For this review, take the finished solid that the model builds, in its own axes (mm). A direction names the side the tool comes from. Coordinates: 2 decimals unless noted, no trailing zeros. Loops run counter-clockwise (first coordinate to the right, second up) from the corner with the lowest first, then second, coordinate; pieces in that order, holes last. Notation, with made-up numbers: (-15.75, 34.25) -> (7.25, 34.25) arc R6 ccw to (7.25, 39.25) -> close; hole circle Ø2 at (-35, 84). An arc over 180 degrees is marked (long way). Use a Markdown table: item, result.
from build123d import *

# Parameters (mm, degrees)
SKETCH_1_R               = 9.8
EXTRUDE_1_DEPTH          = 30
FILLET_1_R               = 0.5
CUT_EXTRUDE_1_DEPTH      = 34.046633746
CUT_EXTRUDE_1_DEPTH_BACK = 34.046633746
CUT_EXTRUDE_START        = -2
SKETCH_5_R               = 8
CUT_EXTRUDE_2_DEPTH      = 23
CHAMFER_1_SIZE           = 0.5
SKETCH_7_R               = 1.5
CUT_EXTRUDE_4_DEPTH      = 7
SKETCH_9_R               = 3
SKETCH_9_R_2             = 1.5
EXTRUDE_2_DEPTH          = 7
CHAMFER_2_SIZE           = 0.5


with BuildPart() as part:
    # Sketch 1 → Extrude 1 (new body)
    with BuildSketch(Plane(origin=(0, 0, 0), x_dir=(1, 0, 0), z_dir=(0, 1, 0))):
        with Locations(Location((0, 0, 0), (0, 0, 270))):
            Circle(SKETCH_1_R)
    extrude(amount=EXTRUDE_1_DEPTH)

    # Fillet 1
    fillet_1_edges = [part.edges().sort_by_distance(p)[0] for p in [
        (0, 30, -9.8),
    ]]
    fillet(fillet_1_edges, radius=FILLET_1_R)

    # Sketch 4 → Cut-Extrude 1 (cut, two sides: drawn at the far end of the back side and taken through both)
    with BuildSketch(Plane.XY.offset(-CUT_EXTRUDE_1_DEPTH_BACK)):
        Polygon((6.75, 3.464101615), (-6.75, 3.464101615), (-8.75, 0), (8.75, 0), align=None)
    extrude(amount=CUT_EXTRUDE_1_DEPTH + CUT_EXTRUDE_1_DEPTH_BACK, mode=Mode.SUBTRACT)

    # Sketch 5 → Cut-Extrude 2 (cut)
    with BuildSketch(Plane.XZ.offset(-3.464101615).offset(CUT_EXTRUDE_START)):
        Circle(SKETCH_5_R)
    extrude(amount=-CUT_EXTRUDE_2_DEPTH, mode=Mode.SUBTRACT)

    # Chamfer 1
    chamfer_1_edges = [part.edges().sort_by_distance(p)[0] for p in [
        (-9.8, 0, 0),
        (9.8, 0, 0),
    ]]
    chamfer(chamfer_1_edges, length=CHAMFER_1_SIZE)

    # Sketch 7 → Cut-Extrude 4 (cut)
    with BuildSketch(Plane.XZ.offset(-3.464101615)):
        with Locations(Location((0, 0, 0), (0, 0, 270))):
            Circle(SKETCH_7_R)
    extrude(amount=-CUT_EXTRUDE_4_DEPTH, mode=Mode.SUBTRACT)

    # Sketch 9 → Extrude 2 (add)
    with BuildSketch(Plane.XZ.offset(-3.464101615)):
        with Locations(Location((0, 0, 0), (0, 0, 270))):
            Circle(SKETCH_9_R)
        with Locations(Location((0, 0, 0), (0, 0, 270))):
            Circle(SKETCH_9_R_2, mode=Mode.SUBTRACT)
    extrude(amount=-EXTRUDE_2_DEPTH)

    # Chamfer 2
    chamfer_2_edges = [part.edges().sort_by_distance(p)[0] for p in [
        (0, 3.464101615, 1.5),
    ]]
    chamfer(chamfer_2_edges, length=CHAMFER_2_SIZE)


solid = part.part
(1) For pin 1 Ø3 at (x, z) = (6.5, 6.5) entering from -Y; pin 2 Ø1.5 at (y, z) = (21, 4.5) entering from +X; pin 3 Ø8 at (x, z) = (1, -2) entering from -Y, all flat-tipped, find the tip position at first contact; note any pin that passes through.
Found:
| item | result |
|---|---|
| pin 1 | stops at y = 1.55 |
| pin 2 | stops at x = 9.05 |
| pin 3 | stops at y = 3.46 |
(2) Take a section at A-A on x = 0. Write out the cut boundary in (y, z).
Found:
| item | result |
|---|---|
| outline | (3.46, -9.8) -> (29.5, -9.8) arc R0.5 ccw to (30, -9.3) -> (30, 9.3) arc R0.5 ccw to (29.5, 9.8) -> (3.46, 9.8) -> (3.46, 2) -> (3.96, 1.5) -> (10.46, 1.5) -> (10.46, 3) -> (5.46, 3) -> (5.46, 8) -> (28.46, 8) -> (28.46, -8) -> (5.46, -8) -> (5.46, -3) -> (10.46, -3) -> (10.46, -1.5) -> (3.96, -1.5) -> (3.46, -2) -> close |
(3) Take a section at C-C on y = 19. Write out the cut boundary in (x, z), plus the area to 3 significant figures.
Found:
| item | result |
|---|---|
| outline | circle Ø19.6 at (0, 0); hole circle Ø16 at (0, 0) |
| area | 101 mm^2 |
(4) Take a section at B-B on z = 0. Write out the cut boundary in (x, y).
Found:
| item | result |
|---|---|
| outline | (-9.8, 0.5) -> (-9.3, 0) -> (-8.75, 0) -> (-6.75, 3.46) -> (-2, 3.46) -> (-1.5, 3.96) -> (-1.5, 10.46) -> (-3, 10.46) -> (-3, 5.46) -> (-8, 5.46) -> (-8, 28.46) -> (8, 28.46) -> (8, 5.46) -> (3, 5.46) -> (3, 10.46) -> (1.5, 10.46) -> (1.5, 3.96) -> (2, 3.46) -> (6.75, 3.46) -> (8.75, 0) -> (9.3, 0) -> (9.8, 0.5) -> (9.8, 29.5) arc R0.5 ccw to (9.3, 30) -> (-9.3, 30) arc R0.5 ccw to (-9.8, 29.5) -> close |
(5) For line 1 along Z through (x, y) = (0, 21); line 2 along Y through (x, z) = (-6.25, 4.25); line 3 along Z through (x, y) = (-2, 7.5), list the stretches that pass through material, from the lowest coordinate up.
Found:
| item | result |
|---|---|
| line 1 | z = -9.8 to -8, 8 to 9.8 |
| line 2 | y = 3.46 to 5.46, 28.46 to 30 |
| line 3 | z = -9.59 to -7.75, -2.24 to 2.24, 7.75 to 9.59 |
(6) Mouldability with a two-part tool opening along Z and no side actions: class faces 1 (the face through (-1.3, 10.464, -1.3)), 2 (the face through (-7.736, 1.756, -0.099)), 3 (the face through (-9.44, 0.14, -0.07)) as pulls with the +Z half, pulls with the -Z half, needs draft (parallel to the pull), parting line crosses it, or undercut.
Found:
| item | result |
|---|---|
| face 1 | undercut |
| face 2 | needs draft |
| face 3 | parting line crosses it |
(7) For faces 4 (the face through (7.764, 1.708, -0.099)), 5 (the face through (0.45, 7.17, -1.43)), 6 (the face through (3.4, 5.464, 0.1)), 7 (the face through (9.44, 0.14, 0.07)), list the 3-axis set-ups (+Z, -Z, +X, -X, +Y, -Y) from which the entire face can be reached by the end or side of a thin tool; tool diameter is ignored.
Found:
| item | result |
|---|---|
| face 4 | +Z, -Z, -Y |
| face 5 | -Y |
| face 6 | none |
| face 7 | +X, -Y |
